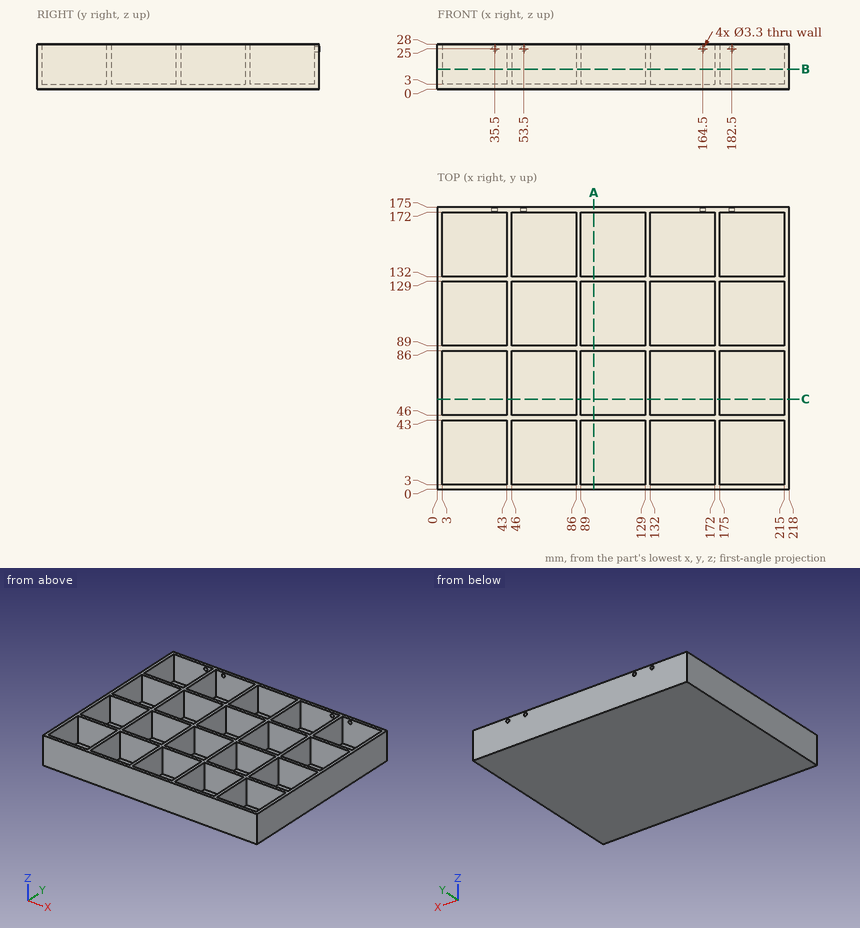
The drawing under review shows one solid part. Ordinate dimensions are in mm from its lowest x, y, z. Round coordinates to 2 decimals unless told otherwise and drop trailing zeros. Loops run counter-clockwise (first coordinate to the right, second up) from the corner with the lowest first, then second, coordinate; pieces in that order, holes last. Notation, with made-up numbers: (45, -19) - (57, -19) arc R16 ccw to (57, 4) - close; hole circle Ø9 at (-7.5, 38). An arc over 180 degrees is marked (long way). One line per item, written item: value. Start each with the question number.
1) Consider section A-A on x = 97. Give the boundary of the cut face in (y, z).
2) Consider section B-B on z = 12.5. Give the number of separate pieces and of enclosed holes in the cut face, then the cut area to 3 significant figures.
3) To check wall thickness, follow L1, parallel to X at y = 111, z = 24.25; L2, parallel to Y at x = 158, z = 18.5; L3, parallel to X at y = 174.25, z = 25. State the ranges of each line that lie inside material, in increasing order. Write a range as from..to.
4) Consider section C-C on y = 56. Give the boundary of the cut face in (x, z), then the cut area to 3 significant figures.
5) Insertion check: pin 1 Ø8 at (x, y) = (58, 141) entering from +Z. The pin has a flat end and moves straight along its axis. Give the tip position at first contact, or say it passes through.
Reported:
1. outline: (0, 0) - (175, 0) - (175, 28) - (172, 28) - (172, 3) - (132, 3) - (132, 28) - (129, 28) - (129, 3) - (89, 3) - (89, 28) - (86, 28) - (86, 3) - (46, 3) - (46, 28) - (43, 28) - (43, 3) - (3, 3) - (3, 28) - (0, 28) - close
2. separate pieces: 1
2. enclosed holes: 20
2. area: 6,150 mm^2
3. L1: x = 0..3, 43..46, 86..89, 129..132, 172..175, 215..218
3. L2: y = 0..3, 43..46, 86..89, 129..132, 172..175
3. L3: x = 0..33.85, 37.15..51.85, 55.15..162.85, 166.15..180.85, 184.15..218
4. outline: (0, 0) - (218, 0) - (218, 28) - (215, 28) - (215, 3) - (175, 3) - (175, 28) - (172, 28) - (172, 3) - (132, 3) - (132, 28) - (129, 28) - (129, 3) - (89, 3) - (89, 28) - (86, 28) - (86, 3) - (46, 3) - (46, 28) - (43, 28) - (43, 3) - (3, 3) - (3, 28) - (0, 28) - close
4. area: 1,100 mm^2
5. pin 1: stops at z = 3
